Source: CAD feature listing. Evaluate the final solid. Frame: model axes, mm. A direction names the side the tool comes from. Round coordinates to 2 decimals unless told otherwise and drop trailing zeros. Loops run counter-clockwise (first coordinate to the right, second up) from the corner with the lowest first, then second, coordinate; pieces in that order, holes last. Notation, with made-up numbers: M 56,50.5 L 69,50.5 A7 ccw 69,54.5 Z; hole C 2.5,-23 d4. An arc over 180 degrees is marked long. One line per item, written item: value.
from build123d import *

# Parameters (mm, degrees)
SKETCH1_R           = 1.65
BOSS_EXTRUDE1_DEPTH = 5
SKETCH2_W           = 1.5
SKETCH2_H           = 3
FILLET1_R           = 0.7
CHAMFER1_SIZE       = 0.5


with BuildPart() as part:
    # Sketch1 → Boss-Extrude1 (new body)
    with BuildSketch(Plane(origin=(0, 0, 0), x_dir=(1, 0, 0), z_dir=(0, 1, 0))):
        with BuildLine():
            ThreePointArc((-6.391530464, 2.787704304), (-10.473118103, 0.400710302), (-7.169117647, -2.981696978))
            ThreePointArc((-7.169117647, -2.981696978), (-5.211302896, -2.794373502), (-3.248717022, -2.666368129))
            ThreePointArc((-3.248717022, -2.666368129), (0, -1), (3.248717022, -2.666368129))
            ThreePointArc((3.248717022, -2.666368129), (5.211302896, -2.794373502), (7.169117647, -2.981696978))
            ThreePointArc((7.169117647, -2.981696978), (10.473118103, 0.400710302), (6.391530464, 2.787704304))
            ThreePointArc((6.391530464, 2.787704304), (4.401545037, 2.367406779), (2.385480795, 2.636064521))
            ThreePointArc((2.385480795, 2.636064521), (0, 3), (-2.385480795, 2.636064521))
            ThreePointArc((-2.385480795, 2.636064521), (-4.401545037, 2.367406779), (-6.391530464, 2.787704304))
        make_face()
        with Locations((-7.5, 0)):
            Circle(SKETCH1_R, mode=Mode.SUBTRACT)
        with Locations((7.5, 0)):
            Circle(SKETCH1_R, mode=Mode.SUBTRACT)
    extrude(amount=BOSS_EXTRUDE1_DEPTH)

    # Sketch2 → Cut-Revolve1 (revolve, cut)
    with BuildSketch(Plane(origin=(0, 0, 0), x_dir=(0, 0, -1), z_dir=(1, 0, 0))):
        with Locations((1.25, 2.5)):
            Rectangle(SKETCH2_W, SKETCH2_H)
    revolve(axis=Axis((0, 0, 5), (0, 1, 0)), mode=Mode.SUBTRACT)

    # Fillet1
    fillet1_edges = [part.edges().sort_by_distance(p)[0] for p in [
        (3.248717022, 2.5, 2.666368129),
        (-3.248717022, 2.5, 2.666368129),
    ]]
    fillet(fillet1_edges, radius=FILLET1_R)

    # Chamfer1
    chamfer1_edges = [part.edges().sort_by_distance(p)[0] for p in [
        (-4.401545037, 0, -2.367406779),
        (0, 0, -3),
        (-9.15, 5, 0),
        (4.401545037, 0, -2.367406779),
        (10.473118103, 0, -0.400710302),
        (-5.369814622, 0, 2.80731824),
        (-10.473118103, 0, -0.400710302),
        (-9.15, 0, 0),
        (5.85, 0, 0),
        (-10.473118103, 5, -0.400710302),
        (-5.369814622, 5, 2.80731824),
        (10.473118103, 5, -0.400710302),
        (4.401545037, 5, -2.367406779),
        (5.369814622, 0, 2.80731824),
        (0, 5, -3),
        (5.369814622, 5, 2.80731824),
        (0, 0, 1),
        (-3.29118131, 0, 2.609929037),
        (3.29118131, 0, 2.609929037),
        (0, 5, 1),
        (-4.401545037, 5, -2.367406779),
        (-3.29118131, 5, 2.609929037),
        (3.29118131, 5, 2.609929037),
        (5.85, 5, 0),
    ]]
    chamfer(chamfer1_edges, length=CHAMFER1_SIZE)


solid = part.part
1. Pull-direction query (X, two-part tool) for faces 4 (the face through (4.543, 2.472, 2.744)), 5 (the face through (0, 5, 0)), 6 (the face through (4.43, 2.47, -2.37)); classes: released by +X, released by -X, zero draft, split by the parting line, or undercut.
Report:
face 4: undercut
face 5: zero draft
face 6: undercut
2. Section query A-A (x = 7.5). Return the cut outline in (y, z), and give its area (3 significant figures).
Report:
outline: M 0,-2.5 L 0.5,-3 L 4.5,-3 L 5,-2.5 L 5,-2.15 L 4.5,-1.65 L 0.5,-1.65 L 0,-2.15 Z; M 0,2.15 L 0.5,1.65 L 4.5,1.65 L 5,2.15 L 5,2.5 L 4.5,3 L 0.5,3 L 0,2.5 Z
area: 12.5 mm2
3. Reachability of faces 1 (the face through (-0.05, 0.36, 0.86)), 2 (the face through (-4.594, 2.472, 2.748)), 3 (the face through (0, 1, -1)) from +Z, -Z, +X, -X, +Y, -Y: full face, straight path, thin tool, end or side. Return the list, or none.
Report:
face 1: +Z, -Y
face 2: +Z, +Y, -Y
face 3: none
4. Ray query, line 1 (X direction, y = 0.65, z = 0); line 2 (X direction, y = 2.6, z = 0); line 3 (Y direction, x = 1.25, z = -1). Return the intervals inside material, ascending. Write a range as [from, to].
Report:
line 1: x = [-10.5, -9.15], [-5.85, 5.85], [9.15, 10.5]
line 2: x = [-10.5, -9.15], [-5.85, -4.9], [-2.29, 2.29], [4.9, 5.85], [9.15, 10.5]
line 3: y = [0, 1], [4, 5]
5. Section query B-B (y = 3.15). Count the separate pieces of the cut face and the enclosed holes in it, and give its area (3 significant figures).
Report:
separate pieces: 2
enclosed holes: 2
area: 62.1 mm2
6. Pin query (flat end, axial travel): pin 1 (2 mm diameter, centred on y = 2, z = -2, fed in from -X); pin 2 (2 mm diameter, centred on x = -7.5, z = 0, fed in from -Y). Return the tip coordinate at first contact, or that it passes through.
Report:
pin 1: stops at x = -10.33
pin 2: passes through
